Design review of the part shown in the three views and the two pictorial views. Dimensions are in mm from the part's minimum x, y and z. Coordinates: 2 decimals unless noted, no trailing zeros. Write each loop counter-clockwise with the first axis right and the second up, starting at its lowest first coordinate (ties: lowest second). Pieces come first, ordered by that corner, then holes. Notation, with made-up numbers: (22.25, 71.25) -> (72.25, 71.25) arc R24 ccw to (72.25, 85.25) -> close; hole circle Ø4 at (34, -37). An arc over 180 degrees is marked (long way). Answer in a Markdown table with one row per item. Add a question column.
Item 1: To check wall thickness, follow line 1 (X direction, y = 18.5, z = 95) (3 decimals); line 2 (X direction, y = 24.15, z = 190.5). State the ranges of each line that lie inside material, in increasing order.
Item 2: Take a section at C-C, the plane x = 12.7. Write out the cut boundary in (y, z) (1 decimal), and give its area (3 significant figures).
Item 3: Draft analysis for pull direction Y (two halves, no side actions). For the marked faces 1, 2 and 3, state which applies: released by +Y, released by -Y, zero draft, split by the parting line, or undercut.
Item 4: Take a section at A-A, the plane y = 12.25. Write out the cut boundary in (x, z) (3 decimals).
Item 5: Take a section at B-B, the plane z = 182.5. Write out the cut boundary in (x, y) (3 decimals), and give its area (3 significant figures).
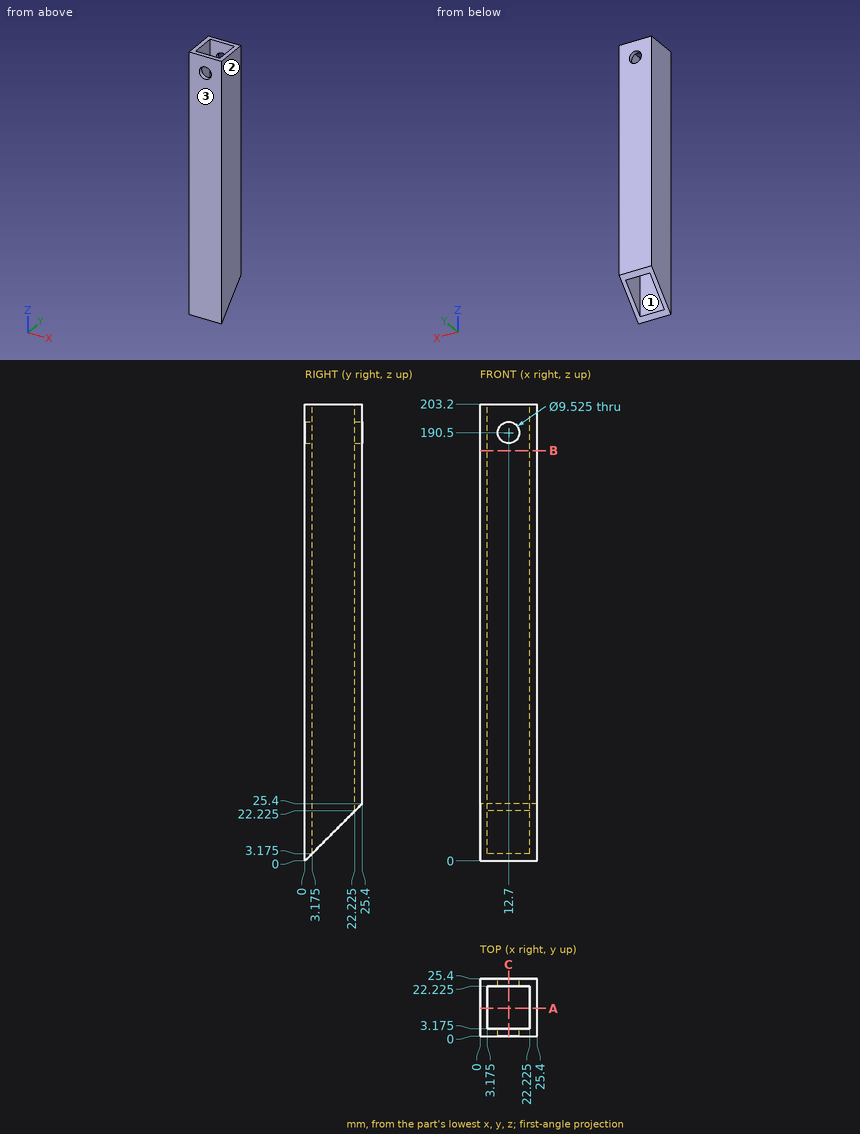
Answers:
| question | item | result |
|---|---|---|
| 1 | line 1 | x = 0 to 3.175, 22.225 to 25.4 |
| 1 | line 2 | x = 0 to 7.94, 17.46 to 25.4 |
| 2 | outline | (0, 0) -> (3.2, 3.2) -> (3.2, 185.7) -> (0, 185.7) -> close; (0, 195.3) -> (3.2, 195.3) -> (3.2, 203.2) -> (0, 203.2) -> close; (22.2, 22.2) -> (25.4, 25.4) -> (25.4, 185.7) -> (22.2, 185.7) -> close; (22.2, 195.3) -> (25.4, 195.3) -> (25.4, 203.2) -> (22.2, 203.2) -> close |
| 2 | area | 1,150 mm^2 |
| 3 | face 1 | undercut |
| 3 | face 2 | zero draft |
| 3 | face 3 | released by -Y |
| 4 | outline | (0, 12.25) -> (3.175, 12.25) -> (3.175, 203.2) -> (0, 203.2) -> close; (22.225, 12.25) -> (25.4, 12.25) -> (25.4, 203.2) -> (22.225, 203.2) -> close |
| 5 | outline | (0, 0) -> (25.4, 0) -> (25.4, 25.4) -> (0, 25.4) -> close; hole (3.175, 3.175) -> (22.225, 3.175) -> (22.225, 22.225) -> (3.175, 22.225) -> close |
| 5 | area | 282 mm^2 |
